Source: CAD feature listing. Evaluate the final solid. Frame: model axes, mm. A direction names the side the tool comes from. Give positions to 0.01 mm unless a question says otherwise; leave off trailing zeros. Order: outer loops, then holes, each group sorted by start corner. A loop starts at its lowest first (then second) coordinate and runs counter-clockwise, first axis right, second up.
from build123d import *

# Parameters (mm, degrees)
F2_DEPTH = 25.4
F2_TAPER = -2
F4_DEPTH = 2.5
F4_TAPER = 2


with BuildPart() as f2:
    # F1 (on Top) → F2 (new body)
    with BuildSketch(Plane.XY):
        with BuildLine():
            Line((-35.6, -31.75), (35.6, -31.75))
            ThreePointArc((35.6, -31.75), (50.8381511346, -25.4381511346), (57.15, -10.2))
            Line((57.15, -10.2), (57.15, 10.2))
            ThreePointArc((57.15, 10.2), (50.8381511346, 25.4381511346), (35.6, 31.75))
            Line((35.6, 31.75), (-35.6, 31.75))
            ThreePointArc((-35.6, 31.75), (-50.8381511346, 25.4381511346), (-57.15, 10.2))
            Line((-57.15, 10.2), (-57.15, -10.2))
            ThreePointArc((-57.15, -10.2), (-50.8381511346, -25.4381511346), (-35.6, -31.75))
        make_face()
        with BuildLine():
            ThreePointArc((54.65, -10.2), (49.0703841816, -23.6703841816), (35.6, -29.25))
            Line((35.6, -29.25), (-35.6, -29.25))
            ThreePointArc((-35.6, -29.25), (-49.0703841816, -23.6703841816), (-54.65, -10.2))
            Line((-54.65, -10.2), (-54.65, 10.2))
            ThreePointArc((-54.65, 10.2), (-49.0703841816, 23.6703841816), (-35.6, 29.25))
            Line((-35.6, 29.25), (35.6, 29.25))
            ThreePointArc((35.6, 29.25), (49.0703841816, 23.6703841816), (54.65, 10.2))
            Line((54.65, 10.2), (54.65, -10.2))
        make_face(mode=Mode.SUBTRACT)
    extrude(amount=F2_DEPTH, taper=F2_TAPER)

    # F3 (on Top) → F4 (join)
    with BuildSketch(Plane.XY):
        with BuildLine():
            Line((-35.6, -31.75), (35.6, -31.75))
            ThreePointArc((35.6, -31.75), (50.8381511346, -25.4381511346), (57.15, -10.2))
            Line((57.15, -10.2), (57.15, 10.2))
            ThreePointArc((57.15, 10.2), (50.8381511346, 25.4381511346), (35.6, 31.75))
            Line((35.6, 31.75), (-35.6, 31.75))
            ThreePointArc((-35.6, 31.75), (-50.8381511346, 25.4381511346), (-57.15, 10.2))
            Line((-57.15, 10.2), (-57.15, -10.2))
            ThreePointArc((-57.15, -10.2), (-50.8381511346, -25.4381511346), (-35.6, -31.75))
        make_face()
    extrude(amount=-F4_DEPTH, taper=F4_TAPER)


solid = f2.part
(1) Access query for faces 1 (the conical face through (48.9, -23.2, 12.9)), 2 (the conical face through (50.94, -25.89, 11.25)). Directions: +Z, -Z, +X, -X, +Y, -Y. A direction counts if a zero-diameter tool reaches every point of the face in a straight line with its end or side. Return the directions, or none.
(2) Section B-B, the plane z = 3.75. Return loops of the section in (x, y).
(3) Section A-A, the plane x = -10. Return loops of the section in (y, z), plus the area to 3 significant figures.
(4) Pin query (flat end, axial travel): pin 1 Ø1.5 at (y, z) = (2.5, 7) entering from +X; pin 2 Ø10 at (x, y) = (-18.5, -22) entering from +Z; pin 3 Ø12 at (y, z) = (11, 15.5) entering from -X. Return the tip coordinate at first contact, or that it passes through.
(5) Draft query along Z for faces 3 (the conical face through (48.6, 23.5, 12.9)), 4 (the conical face through (-50.94, 25.89, 11.25)), 5 (the flat face through (0, 29, 25.4)). Return one class per face: +Z half, -Z half, draft (parallel to the pull), parting line (faces both ways), or undercut.
(6) Section D-D, the plane z = 21.25. Return loops of the section in (x, y), plus the area to 3 significant figures.
(7) Line query: line 1 along Z through (x, y) = (-0.5, 19); line 2 along X through (y, z) = (-7, 16.75); line 3 along X through (y, z) = (-15, 8). Output: solid intervals per line, ascending.
(8) Section C-C, the plane y = -2. Return loops of the section in (x, z).
Checks:
1. face 1: none
1. face 2: -Z, +X, -Y
2. outline: (-57.28, -10.2) arc R21.68 ccw to (-35.6, -31.88) - (35.6, -31.88) arc R21.68 ccw to (57.28, -10.2) - (57.28, 10.2) arc R21.68 ccw to (35.6, 31.88) - (-35.6, 31.88) arc R21.68 ccw to (-57.28, 10.2) - close; hole (-54.52, -10.2) arc R18.92 ccw to (-35.6, -29.12) - (35.6, -29.12) arc R18.92 ccw to (54.52, -10.2) - (54.52, 10.2) arc R18.92 ccw to (35.6, 29.12) - (-35.6, 29.12) arc R18.92 ccw to (-54.52, 10.2) - close
3. outline: (-32.64, 25.4) - (-31.66, -2.5) - (31.66, -2.5) - (32.64, 25.4) - (28.36, 25.4) - (29.25, 0) - (-29.25, 0) - (-28.36, 25.4) - close
3. area: 331 mm2
4. pin 1: stops at x = 57.42
4. pin 2: stops at z = 0
4. pin 3: stops at x = -57.9
5. face 3: undercut
5. face 4: -Z half
5. face 5: +Z half
6. outline: (-57.89, -10.2) arc R22.29 ccw to (-35.6, -32.49) - (35.6, -32.49) arc R22.29 ccw to (57.89, -10.2) - (57.89, 10.2) arc R22.29 ccw to (35.6, 32.49) - (-35.6, 32.49) arc R22.29 ccw to (-57.89, 10.2) - close; hole (-53.91, -10.2) arc R18.31 ccw to (-35.6, -28.51) - (35.6, -28.51) arc R18.31 ccw to (53.91, -10.2) - (53.91, 10.2) arc R18.31 ccw to (35.6, 28.51) - (-35.6, 28.51) arc R18.31 ccw to (-53.91, 10.2) - close
6. area: 1,240 mm2
7. line 1: z = -2.5 to 0
7. line 2: x = -57.73 to -54.07, 54.07 to 57.73
7. line 3: x = -56.9 to -53.75, 53.75 to 56.9
8. outline: (-58.04, 25.4) - (-57.06, -2.5) - (57.06, -2.5) - (58.04, 25.4) - (53.76, 25.4) - (54.65, 0) - (-54.65, 0) - (-53.76, 25.4) - close
